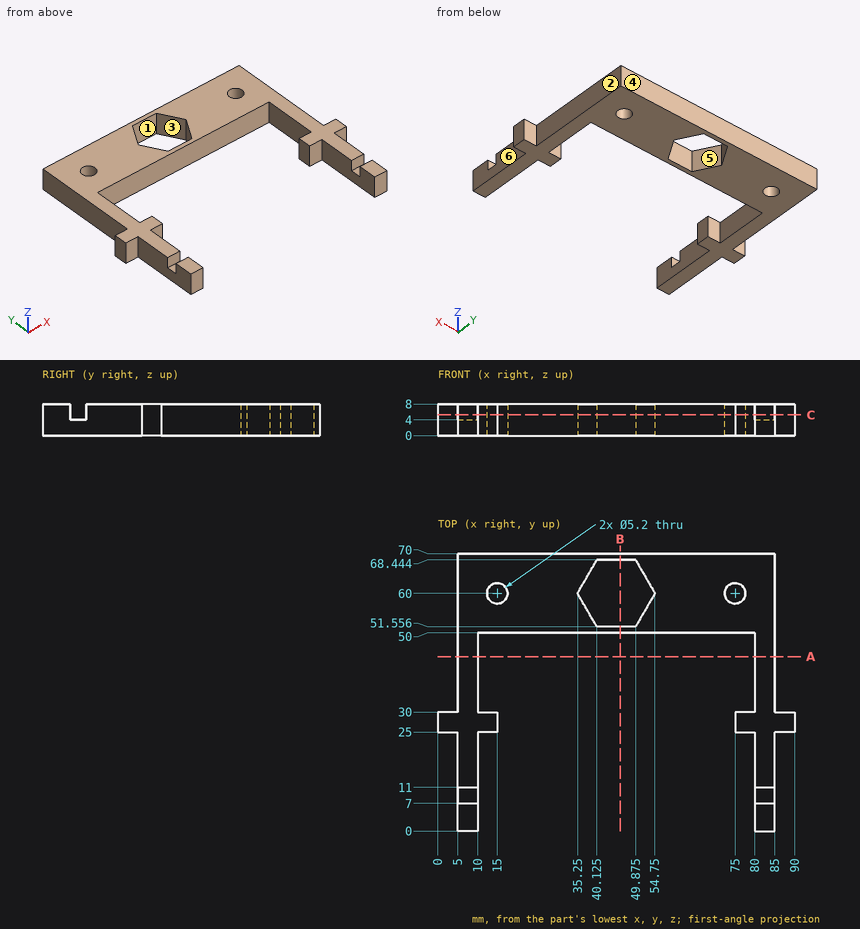
For this review, use the dimensioned drawing (mm, ordinates from the lowest corner) and the shaded views. A direction names the side the tool comes from. Give positions to 0.01 mm unless a question says otherwise; leave off trailing zeros. Write each loop counter-clockwise with the first axis right and the second up, starting at its lowest first coordinate (ties: lowest second). Pieces come first, ordered by that corner, then holes. Notation, with made-up numbers: M 26.5,-8.5 L 42.5,-8.5 A25 cw 42.5,22.5 Z; hole C 57,-37.75 d1. An arc over 180 degrees is marked long. Answer as a JSON object with one key per item and string values. Group by question number.
Item 1: Consider section B-B on x = 46. Write out the cut boundary in (y, z).
Item 2: For probe 1 along X at (y, z) = (60, 5.75); probe 2 along Y at (x, z) = (11, 2.5); probe 3 along X at (y, z) = (62, 6.25) (1 decimal), list the stretches that pass through material, from the lowest coordinate up. Write a range as [from, to].
Item 3: Consider section C-C on z = 5.25. Count the separate pieces of the cut face and the enclosed holes in it, plus the area to 3 significant figures.
Item 4: Tool access review of the marked faces 5 and 6: name each direction out of +Z, -Z, +X, -X, +Y, -Y from which nothing blocks a thin tool from reaching the whole face with its end or side.
Item 5: Draft analysis for pull direction X (two halves, no side actions). For the marked faces 1, 2, 3 and 4, state which applies: +X half, -X half, draft (parallel to the pull), parting line (faces both ways), or undercut.
Item 6: For pin 1 Ø3 at (x, z) = (81.5, 5.5) entering from -Y; pin 2 Ø4 at (x, z) = (29.5, 2) entering from -Y; pin 3 Ø4 at (y, z) = (43.5, 5) entering from +X; pin 4 Ø2.5 at (y, z) = (47, 6) entering from -X, all flat-tipped, find the tip position at first contact; note any pin that passes through.
Item 7: Consider section A-A on y = 44. Write out the cut boundary in (x, z), plus the area to 3 significant figures.
Check result:
{
 "1": {"outline": "M 50,0 L 51.56,0 L 51.56,8 L 50,8 Z; M 68.44,0 L 70,0 L 70,8 L 68.44,8 Z"},
 "2": {"probe 1": "x = [5, 12.4], [17.6, 35.25], [54.75, 72.4], [77.6, 85]", "probe 2": "y = [25, 30], [50, 70]", "probe 3": "x = [5, 13.3], [16.7, 36.4], [53.6, 73.3], [76.7, 85]"},
 "3": {"separate pieces": "3", "enclosed holes": "3", "area": "1,870 mm^2"},
 "4": {"face 5": "+Z, -Z", "face 6": "+Z, -Z, +X, -Y"},
 "5": {"face 1": "undercut", "face 2": "+X half", "face 3": "undercut", "face 4": "draft"},
 "6": {"pin 1": "stops at y = 0", "pin 2": "stops at y = 50", "pin 3": "stops at x = 85", "pin 4": "stops at x = 5"},
 "7": {"outline": "M 5,0 L 10,0 L 10,8 L 5,8 Z; M 80,0 L 85,0 L 85,8 L 80,8 Z", "area": "80.0 mm^2"}
}
